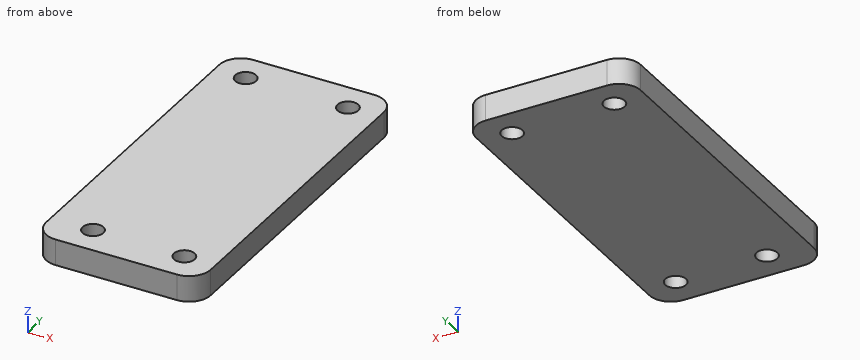
from build123d import *

# Parameters (mm, degrees)
SKETCH1_W            = 38
SKETCH1_H            = 81
BOSS_EXTRUDE1_DEPTH  = 6
M4_CLEARANCE_HOLE1_D = 4.8
FILLET1_R            = 5


with BuildPart() as part:
    # Sketch1 → Boss-Extrude1 (new body)
    with BuildSketch(Plane.XY):
        Rectangle(SKETCH1_W, SKETCH1_H)
    extrude(amount=BOSS_EXTRUDE1_DEPTH)

    # M4 Clearance Hole1 (through all)
    with Locations(Plane.XY.offset(6)):
        with Locations((-11.80805, 33.54195), (11.80805, 33.54195), (11.80805, -33.54195), (-9.28425, -33.54195)):
            Hole(M4_CLEARANCE_HOLE1_D / 2)

    # Fillet1
    fillet1_edges = [part.edges().sort_by_distance(p)[0] for p in [
        (19, -40.5, 3),
        (-19, -40.5, 3),
        (-19, 40.5, 3),
        (19, 40.5, 3),
    ]]
    fillet(fillet1_edges, radius=FILLET1_R)


solid = part.part
Can you work these out from the model? Positions are in its coordinate system, mm. Round coordinates to 2 decimals unless told otherwise and drop trailing zeros. Write each loop counter-clockwise with the first axis right and the second up, starting at its lowest first coordinate (ties: lowest second). Pieces come first, ordered by that corner, then holes. Notation, with made-up numbers: (79, 24.25) -> (89, 24.25) arc R9 ccw to (89, 38.25) -> close; hole circle Ø1 at (81.5, -35.5). An arc over 180 degrees is marked (long way). One line per question, with ' | ' between items. Start each with the question number.
1) I need wall thicknesses on line 1 (X direction, y = 34.5, z = 1.65); line 2 (Y direction, x = -10.5, z = 0.8); line 3 (X direction, y = -34.5, z = 1.1). Which ranges of each line are inside material? Lowest first, please. Write a range as [from, to].
2) Suppose I cut it at C-C on x = 11.5. Write out the boundary of the cut face in (y, z), then the cut area to 3 significant figures.
3) Suppose I cut it at B-B on z = 1.45. Write out the boundary of the cut face in (x, y), then the cut area to 3 significant figures.
4) Suppose I cut it at A-A on x = -13. Write out the boundary of the cut face in (y, z).
5) I'm going to push a flat-ended pin straight in: P1, Ø3, axis at x = -9.28, y = -33.54, coming from the -Z side. Where does the tip first touch, or does it pass through?
Return value:
1) line 1: x = [-19, -14.01], [-9.61, 9.61], [14.01, 19] | line 2: y = [-40.5, -35.61], [-31.47, 31.53], [35.55, 40.5] | line 3: x = [-19, -11.48], [-7.08, 9.61], [14.01, 19]
2) outline: (-40.5, 0) -> (-35.92, 0) -> (-35.92, 6) -> (-40.5, 6) -> close; (-31.16, 0) -> (31.16, 0) -> (31.16, 6) -> (-31.16, 6) -> close; (35.92, 0) -> (40.5, 0) -> (40.5, 6) -> (35.92, 6) -> close | area: 429 mm2
3) outline: (-19, -35.5) arc R5 ccw to (-14, -40.5) -> (14, -40.5) arc R5 ccw to (19, -35.5) -> (19, 35.5) arc R5 ccw to (14, 40.5) -> (-14, 40.5) arc R5 ccw to (-19, 35.5) -> close; hole circle Ø4.8 at (-11.81, 33.54); hole circle Ø4.8 at (-9.28, -33.54); hole circle Ø4.8 at (11.81, -33.54); hole circle Ø4.8 at (11.81, 33.54) | area: 2,980 mm2
4) outline: (-40.5, 0) -> (31.46, 0) -> (31.46, 6) -> (-40.5, 6) -> close; (35.63, 0) -> (40.5, 0) -> (40.5, 6) -> (35.63, 6) -> close
5) P1: passes through
